Could you check a few things on this drawing? It's one solid part, dimensions in mm from its lowest x, y, z. A direction names the side the tool comes from. Give positions to 0.01 mm unless a question says otherwise; leave off trailing zeros. Loops run counter-clockwise (first coordinate to the right, second up) from the corner with the lowest first, then second, coordinate; pieces in that order, holes last. Notation, with made-up numbers: (-2.5, 40) - (13.5, 40) arc R5 cw to (13.5, 44) - close; hole circle Ø7 at (18, 33.25). An arc over 180 degrees is marked (long way). Put each result on its own line as item: value. Start each with the question number.
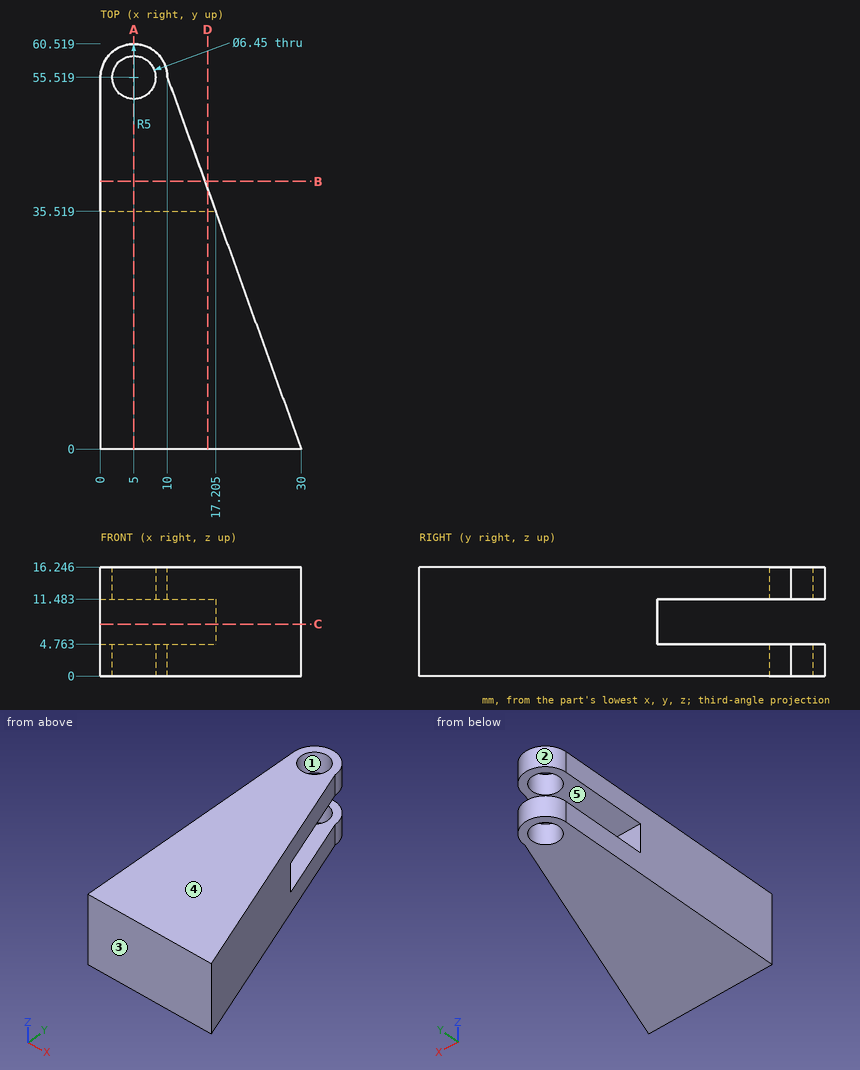
1) Suppose I cut it at A-A on x = 5. Please give me the cut outline in (y, z) (1 decimal).
2) Which directions (+Z, -Z, +X, -X, +Y, -Y) give clear straight access to the entire face, cutting with the end or side of a thin tool? Please do the marked faces 4 and 5.
3) Suppose I cut it at C-C on z = 7.75. Please give me the cut outline in (x, y) (1 decimal).
4) I need wall thicknesses on line 1 (Y direction, x = 5, z = 2.2); line 2 (Y direction, x = 8.5, z = 10.75); line 3 (X direction, y = 56, z = 3.5). Which ranges of each line are inside material? Lowest first, please.
5) I'm going to push flat-ended pins straight in: P1, Ø7.5, axis at x = 4.5, z = 9, coming from the +Y side; P2, Ø5, axis at x = 5, y = 55.52, coming from the +Z side. Where does each tip first touch, or does it pass through?
6) Thinking about a two-plate mould opening in X: for the marked faces 1, 2 and 3, which applies, pulls with the +X half, pulls with the -X half, needs draft (parallel to the pull), parting line crosses it, or undercut?
7) Suppose I cut it at B-B on y = 40. Please give me the cut outline in (x, z) (1 decimal).
8) Suppose I cut it at D-D on x = 16. Please give me the cut outline in (y, z) (1 decimal).
Ans:
1. outline: (0, 0) - (52.3, 0) - (52.3, 4.8) - (35.5, 4.8) - (35.5, 11.5) - (52.3, 11.5) - (52.3, 16.2) - (0, 16.2) - close; (58.7, 0) - (60.5, 0) - (60.5, 4.8) - (58.7, 4.8) - close; (58.7, 11.5) - (60.5, 11.5) - (60.5, 16.2) - (58.7, 16.2) - close
2. face 4: +Z, +X, -X, +Y, -Y
2. face 5: +X, -X, +Y
3. outline: (0, 0) - (30, 0) - (17.2, 35.5) - (0, 35.5) - close
4. line 1: y = 0 to 52.29, 58.74 to 60.52
4. line 2: y = 0 to 35.52
4. line 3: x = 0.02 to 1.81, 8.19 to 9.98
5. P1: stops at y = 60.52
5. P2: passes through
6. face 1: undercut
6. face 2: parting line crosses it
6. face 3: needs draft
7. outline: (0, 0) - (15.6, 0) - (15.6, 4.8) - (0, 4.8) - close; (0, 11.5) - (15.6, 11.5) - (15.6, 16.2) - (0, 16.2) - close
8. outline: (0, 0) - (38.9, 0) - (38.9, 4.8) - (35.5, 4.8) - (35.5, 11.5) - (38.9, 11.5) - (38.9, 16.2) - (0, 16.2) - close
